For this review, take the finished solid that the model builds, in its own axes (mm). A direction names the side the tool comes from. Coordinates: 2 decimals unless noted, no trailing zeros. Write each loop counter-clockwise with the first axis right and the second up, starting at its lowest first coordinate (ties: lowest second). Pieces come first, ordered by that corner, then holes.
1) To check wall thickness, follow line 1 along Y through (x, z) = (0, -3.75); line 2 along Y through (x, z) = (-18, -1.5); line 3 along X through (y, z) = (-393, -7.75). State the ranges of each line that lie inside material, in increasing order.
2) Mouldability with a two-part tool opening along X and no side actions: class faces 4 (the face through (-90.27, -454.43, -8.11)), 5 (the face through (-26, -195, -16)), 6 (the face through (-205.087, -125.138, -8.112)) as pulls with the +X half, pulls with the -X half, needs draft (parallel to the pull), parting line crosses it, or undercut.
3) We need section D-D on y = -190. Write out the cut boundary in (x, z), then the cut area to 3 significant figures.
4) We need section A-A on y = -29. Write out the cut boundary in (x, z).
5) For faces 1 (the face through (220.163, -75.161, -7.888)), 2 (the face through (94.847, -270.509, -8.112)), 3 (the face through (203.66, -241.36, -7.89)), list the 3-axis set-ups (+Z, -Z, +X, -X, +Y, -Y) from which the entire face can be reached by the end or side of a thin tool; tool diameter is ignored.
6) We need section C-C on x = -229. Write out the cut boundary in (y, z).
7) Insertion check: P1, Ø5, axis at x = 80.5, z = -11.5, coming from the +Y side; P2, Ø8, axis at y = -298, z = -4.5, coming from the +X side; P3, Ø1.5, axis at y = -233, z = -6, coming from the +X side. Each pin has a flat end and moves straight along its axis. Give the tip position at first contact, or say it passes through.
8) We need section B-B on y = -129.5. Write out the cut boundary in (x, z), then the cut area to 3 significant figures.
from build123d import *

# Parameters (mm, degrees)
ESTRUSIONE_ESTRUSIONE1_DEPTH  = 16
SCHIZZO3_R                    = 36
TAGLIO_ESTRUSIONE1_DEPTH      = 597.553643858
TAGLIO_ESTRUSIONE4_DEPTH      = 597.553643858
TAGLIO_ESTRUSIONE4_DEPTH_BACK = 597.553643858
RACCORDO2_R                   = 10
TAGLIO_ESTRUSIONE16_DEPTH     = 597.553643858
RACCORDO3_R                   = 30
SCHIZZO39_W                   = 120
SCHIZZO39_H                   = 180
TAGLIO_ESTRUSIONE25_DEPTH     = 597.553643858
RACCORDO5_R                   = 10
TAGLIO_ESTRUSIONE26_DEPTH     = 597.553643858
RACCORDO6_R                   = 10
RACCORDO7_R                   = 30
M6_CLEARANCE_HOLE1_D          = 6.6
RIPETIZIONE_A_L3_COUNT        = 2
RIPETIZIONE_A_L3_PITCH        = 54
RIPETIZIONE_A_L3_COUNT_DIR2   = 2
RIPETIZIONE_A_L3_PITCH_DIR2   = 129
F_6_0_6_DIAMETER_HOLE2_D      = 6
RIPETIZIONE_A_L4_COUNT        = 2
RIPETIZIONE_A_L4_PITCH        = 54
F_11_0_11_DIAMETER_HOLE1_D    = 11
RIPETIZIONE_A_L5_COUNT        = 2
RIPETIZIONE_A_L5_PITCH        = 190
RIPETIZIONE_A_L5_COUNT_DIR2   = 2
RIPETIZIONE_A_L5_PITCH_DIR2   = 175
M5_CLEARANCE_HOLE1_D          = 5.5
RIPETIZIONECIRCOLARE1_COUNT   = 3
SPECCHIA7_COPY_1_D            = 5.5
SPECCHIA7_COPY_2_D            = 5.5


# Read off the part's stored shape, not the designer's step: Specchia8
with BuildPart() as part:
    # Schizzo2 → Estrusione-Estrusione1 (new body)
    with BuildSketch(Plane.XY):
        with BuildLine():
            Line((-330, 0), (330, 0))
            ThreePointArc((330, 0), (377.167935033, -34.485476873), (358.614305107, -89.891478597))
            ThreePointArc((358.614305107, -89.891478597), (195.466897987, -252.623261021), (95, -460))
            Line((95, -460), (-95, -460))
            ThreePointArc((-95, -460), (-195.466897987, -252.623261021), (-358.614305107, -89.891478597))
            ThreePointArc((-358.614305107, -89.891478597), (-377.167935033, -34.485476873), (-330, 0))
        make_face()
    extrude(amount=-ESTRUSIONE_ESTRUSIONE1_DEPTH)

    # Schizzo3 → Taglio-Estrusione1 (cut, symmetric)
    with BuildSketch(Plane.XY):
        with Locations((-330, -49.5)):
            Circle(SCHIZZO3_R)
    taglio_estrusione1 = extrude(amount=TAGLIO_ESTRUSIONE1_DEPTH, both=True, mode=Mode.SUBTRACT)

    # Specchia1: Taglio-Estrusione1 across plane
    add(taglio_estrusione1.mirror(Plane(origin=(0, 0, 0), x_dir=(0, 0, 1), z_dir=(1, 0, 0))), mode=Mode.SUBTRACT)

    # Schizzo12 → Taglio-Estrusione4 (cut, two sides: drawn at the far end of the back side and taken through both)
    with BuildSketch(Plane(origin=(0, 0, -16), x_dir=(-1, 0, 0), z_dir=(0, 0, -1)).offset(-TAGLIO_ESTRUSIONE4_DEPTH_BACK)):
        with BuildLine():
            Line((-330, 0), (330, 0))
            ThreePointArc((330, 0), (314.985476873, -2.332064967), (301.385694893, -9.108521403))
            ThreePointArc((301.385694893, -9.108521403), (216.113325417, -78.953204124), (141.406742184, -160))
            Line((141.406742184, -160), (36, -160))
            Line((36, -160), (36, -107.15))
            Line((36, -107.15), (-36, -107.15))
            Line((-36, -107.15), (-36, -160))
            Line((-36, -160), (-141.406742184, -160))
            ThreePointArc((-141.406742184, -160), (-216.113325417, -78.953204124), (-301.385694893, -9.108521403))
            ThreePointArc((-301.385694893, -9.108521403), (-314.985476873, -2.332064967), (-330, 0))
        make_face()
    extrude(amount=TAGLIO_ESTRUSIONE4_DEPTH + TAGLIO_ESTRUSIONE4_DEPTH_BACK, mode=Mode.SUBTRACT)

    # Raccordo2
    raccordo2_edges = [part.edges().sort_by_distance(p)[0] for p in [
        (36, -160, -8),
        (36, -107.15, -8),
        (-36, -160, -8),
        (-36, -107.15, -8),
    ]]
    fillet(raccordo2_edges, radius=RACCORDO2_R)

    # Schizzo24 → Taglio-Estrusione16 (cut, through all)
    with BuildSketch(Plane(origin=(0, 0, -16), x_dir=(-1, 0, 0), z_dir=(0, 0, -1))):
        with BuildLine():
            ThreePointArc((200.293142061, -204.853472831), (239.934023772, -159.597976721), (283.239119921, -117.835217253))
            ThreePointArc((283.239119921, -117.835217253), (285.324112305, -83.249775131), (250.738670183, -81.164782747))
            ThreePointArc((250.738670183, -81.164782747), (204.4658122, -125.789605452), (162.108282651, -174.146527169))
            ThreePointArc((162.108282651, -174.146527169), (165.847239525, -208.592429705), (200.293142061, -204.853472831))
        make_face()
    taglio_estrusione16 = extrude(amount=-TAGLIO_ESTRUSIONE16_DEPTH, mode=Mode.SUBTRACT)

    # Specchia3: Taglio-Estrusione16 across plane
    add(taglio_estrusione16.mirror(Plane(origin=(0, 0, 0), x_dir=(0, 0, 1), z_dir=(1, 0, 0))), mode=Mode.SUBTRACT)

    # Raccordo3
    raccordo3_edges = [part.edges().sort_by_distance(p)[0] for p in [
        (-141.406742184, -160, -8),
        (141.406742184, -160, -8),
        (-95, -460, -8),
        (95, -460, -8),
    ]]
    fillet(raccordo3_edges, radius=RACCORDO3_R)

    # Schizzo39 → Taglio-Estrusione25 (cut, through all)
    with BuildSketch(Plane(origin=(0, 0, -16), x_dir=(-1, 0, 0), z_dir=(0, 0, -1))):
        with Locations((0, -290)):
            Rectangle(SCHIZZO39_W, SCHIZZO39_H)
    extrude(amount=-TAGLIO_ESTRUSIONE25_DEPTH, mode=Mode.SUBTRACT)

    # Raccordo5
    raccordo5_edges = [part.edges().sort_by_distance(p)[0] for p in [
        (60, -380, -8),
        (60, -200, -8),
        (-60, -200, -8),
        (-60, -380, -8),
    ]]
    fillet(raccordo5_edges, radius=RACCORDO5_R)

    # Schizzo40 → Taglio-Estrusione26 (cut, through all)
    with BuildSketch(Plane(origin=(0, 0, -16), x_dir=(-1, 0, 0), z_dir=(0, 0, -1))):
        with BuildLine():
            Line((165, -261.686426461), (110, -220))
            Line((110, -220), (80, -320))
            Line((80, -320), (106.286172484, -370))
            ThreePointArc((106.286172484, -370), (133.289241422, -314.567258295), (165, -261.686426461))
        make_face()
    taglio_estrusione26 = extrude(amount=-TAGLIO_ESTRUSIONE26_DEPTH, mode=Mode.SUBTRACT)

    # Specchia6: Taglio-Estrusione26 across plane
    add(taglio_estrusione26.mirror(Plane(origin=(0, 0, 0), x_dir=(0, 0, 1), z_dir=(1, 0, 0))), mode=Mode.SUBTRACT)

    # Raccordo6
    raccordo6_edges = [part.edges().sort_by_distance(p)[0] for p in [
        (-165, -261.686426461, -8),
        (-106.286172484, -370, -8),
        (-110, -220, -8),
        (106.286172484, -370, -8),
        (165, -261.686426461, -8),
        (110, -220, -8),
    ]]
    fillet(raccordo6_edges, radius=RACCORDO6_R)

    # Raccordo7
    raccordo7_edges = [part.edges().sort_by_distance(p)[0] for p in [
        (-80, -320, -8),
        (80, -320, -8),
    ]]
    fillet(raccordo7_edges, radius=RACCORDO7_R)

    # M6 Clearance Hole1 (through all)
    with Locations(Plane(origin=(0, 0, -16), x_dir=(-1, 0, 0), z_dir=(0, 0, -1))):
        with Locations((64.5, -393)):
            m6_clearance_hole1 = Hole(M6_CLEARANCE_HOLE1_D / 2)

    # Ripetizione a L3: M6 Clearance Hole1 2 × 2
    with Locations(*[(j * RIPETIZIONE_A_L3_PITCH_DIR2, -i * RIPETIZIONE_A_L3_PITCH, 0) for i in range(RIPETIZIONE_A_L3_COUNT) for j in range(RIPETIZIONE_A_L3_COUNT_DIR2) if (i, j) != (0, 0)]):
        add(m6_clearance_hole1, mode=Mode.SUBTRACT)

    # Ø6.0 (6) Diameter Hole2 (through all)
    with Locations(Plane(origin=(0, 0, -16), x_dir=(-1, 0, 0), z_dir=(0, 0, -1))):
        with Locations((0, -393)):
            f_6_0_6_diameter_hole2 = Hole(F_6_0_6_DIAMETER_HOLE2_D / 2)

    # Ripetizione a L4: Ø6.0 (6) Diameter Hole2 ×2
    with Locations(*[(0, -i * RIPETIZIONE_A_L4_PITCH, 0) for i in range(1, RIPETIZIONE_A_L4_COUNT)]):
        add(f_6_0_6_diameter_hole2, mode=Mode.SUBTRACT)

    # Ø11.0 (11) Diameter Hole1 (through all)
    with Locations(Plane.XY):
        with Locations((-95, -213)):
            f_11_0_11_diameter_hole1 = Hole(F_11_0_11_DIAMETER_HOLE1_D / 2)

    # Ripetizione a L5: 11.0 _11_ Diameter Hole1 2 × 2
    with Locations(*[(i * RIPETIZIONE_A_L5_PITCH, -j * RIPETIZIONE_A_L5_PITCH_DIR2, 0) for i in range(RIPETIZIONE_A_L5_COUNT) for j in range(RIPETIZIONE_A_L5_COUNT_DIR2) if (i, j) != (0, 0)]):
        add(f_11_0_11_diameter_hole1, mode=Mode.SUBTRACT)

    # M5 Clearance Hole1 (through all)
    with Locations(Plane.XY):
        with Locations((-372, -49.5)):
            m5_clearance_hole1 = Hole(M5_CLEARANCE_HOLE1_D / 2)

    # RipetizioneCircolare1: M5 Clearance Hole1 ×3 about axis
    ripetizionecircolare1_axis = Axis((-330, -49.5, 0), (0, 0, 1))
    for i in range(1, RIPETIZIONECIRCOLARE1_COUNT):
        add(m5_clearance_hole1.rotate(ripetizionecircolare1_axis, i * 360 / RIPETIZIONECIRCOLARE1_COUNT), mode=Mode.SUBTRACT)

    # Specchia7: M5 Clearance Hole1 across plane
    add(m5_clearance_hole1.mirror(Plane(origin=(0, 0, 0), x_dir=(0, 0, 1), z_dir=(1, 0, 0))), mode=Mode.SUBTRACT)

    # Specchia7 copy 1 (through all)
    with Locations(Plane(origin=(537.868257487, 211.538383249, 0), x_dir=(0.4999999999999998, 0.8660254037844387, 0), z_dir=(0, 0, 1))):
        with Locations((-372, 49.5)):
            Hole(SPECCHIA7_COPY_1_D / 2)

    # Specchia7 copy 2 (through all)
    with Locations(Plane(origin=(452.131742513, -360.038383249, 0), x_dir=(0.5000000000000004, -0.8660254037844384, 0), z_dir=(0, 0, 1))):
        with Locations((-372, 49.5)):
            Hole(SPECCHIA7_COPY_2_D / 2)

    # Specchia8: part across plane


with BuildPart() as part_1:
    add(part.part)
    add(part.part.mirror(Plane(origin=(0, 0, 0), x_dir=(0, 0, 1), z_dir=(1, 0, 0))))


solid = part_1.part
Result:
1. line 1: y = -460 to -450, -444 to -396, -390 to -380, -200 to -107.15
1. line 2: y = -460 to -380, -200 to -107.15
1. line 3: x = -118.31 to -97.29, -92.71 to -67.8, -61.2 to -3, 3 to 61.2, 67.8 to 92.71, 97.29 to 118.31
2. face 4: pulls with the -X half
2. face 5: needs draft
2. face 6: undercut
3. outline: (-245.82, -16) - (-212.57, -16) - (-212.57, 0) - (-245.82, 0) - close; (-156.71, -16) - (156.71, -16) - (156.71, 0) - (-156.71, 0) - close; (212.57, -16) - (245.82, -16) - (245.82, 0) - (212.57, 0) - close
3. area: 6,080 mm2
4. outline: (-375.06, -16) - (-359.59, -16) - (-359.59, 0) - (-375.06, 0) - close; (-300.41, -16) - (-274.53, -16) - (-274.53, 0) - (-300.41, 0) - close; (274.53, -16) - (300.41, -16) - (300.41, 0) - (274.53, 0) - close; (359.59, -16) - (375.06, -16) - (375.06, 0) - (359.59, 0) - close
5. face 1: +Z, -Z, +Y
5. face 2: +Z, -Z
5. face 3: +Z, -Z, +X, -Y
6. outline: (-209.29, -16) - (-171.33, -16) - (-171.33, 0) - (-209.29, 0) - close; (-101.2, -16) - (-67.07, -16) - (-67.07, 0) - (-101.2, 0) - close
7. P1: stops at y = -160
7. P2: stops at x = 168.18
7. P3: stops at x = 210.55
8. outline: (-307.89, -16) - (-270.4, -16) - (-270.4, 0) - (-307.89, 0) - close; (-200.95, -16) - (-167.1, -16) - (-167.1, 0) - (-200.95, 0) - close; (-36, -16) - (36, -16) - (36, 0) - (-36, 0) - close; (167.1, -16) - (200.95, -16) - (200.95, 0) - (167.1, 0) - close; (270.4, -16) - (307.89, -16) - (307.89, 0) - (270.4, 0) - close
8. area: 3,440 mm2
